Read the model definition and answer for the solid it produces. Units are mm, in the model's axes. A direction names the side the tool comes from. Give positions to 0.01 mm unless a question says otherwise; leave off trailing zeros. Order: outer loops, then holes, each group sorted by start corner. A loop starts at its lowest first (then second) coordinate and runs counter-clockwise, first axis right, second up. Notation, with made-up numbers: (5.5, -4) - (37.5, -4) arc R25 ccw to (37.5, 20) - close; hole circle Ø1 at (-25, -0.75). An arc over 180 degrees is marked (long way). Use a Markdown table: item, result. Add a question column.
1. Flat-ended cylindrical pins translate along their axes: P1, Ø6, axis at y = -3.5, z = 12.5, coming from the -X side; P2, Ø1.5, axis at x = 5, z = 33.5, coming from the -Y side; P3, Ø1.2, axis at y = 0, z = 114.5, coming from the +X side. Find the tip coordinate at first contact, or state that the pin passes through.
2. A cutting plane is placed at D-D on z = 97. Determine the outline of the cut face in (x, y), and give its area (3 significant figures).
3. For a pull along Y with two mould halves and no side action, classify faces 5 (the flat face through (0, 0, 90)), 6 (the flat face through (0, 0, 120)), 7 (the cylindrical face through (-1.5, -0.07, 44.37)), 8 (the flat face through (0, -2, 110)) as released by +Y, released by -Y, zero draft, split by the parting line, or undercut.
4. A cutting plane is placed at A-A on x = 0. Determine the outline of the cut face in (y, z), and give its area (3 significant figures).
5. Which of the six approach directions +Z, -Z, +X, -X, +Y, -Y give full straight-line access (tool end or side, diameter ignored) to faces 1 (the flat face through (2, 0, 110)), 2 (the flat face through (0, 2, 110)), 3 (the cylindrical face through (-1.08, -4.88, 51.33)), 4 (the flat face through (-2, 0, 110))?
6. Consider L1, parallel to Y at x = 0, z = 64.5; L2, parallel to Z at x = -6.5, y = 1. Determine where each line is inside the solid, lowest interval first.
7. A cutting plane is placed at C-C on z = 37.5. Determine the outline of the cut face in (x, y).
```python
from build123d import *

# Parameters (mm, degrees)
F0_R     = 7.5
F1_DEPTH = 4
F2_R     = 5
F3_DEPTH = 100
F4_W     = 4
F4_H     = 4
F5_DEPTH = 20
F6_R     = 1.5
F7_DEPTH = 90


with BuildPart() as f1:
    # F0 (on Top) → F1 (new body)
    with BuildSketch(Plane.XY):
        Circle(F0_R)
    extrude(amount=F1_DEPTH)

    # F2 (on Top) → F3 (join)
    with BuildSketch(Plane.XY):
        Circle(F2_R)
    extrude(amount=F3_DEPTH)

    # F4 (on face) → F5 (join)
    with BuildSketch(Plane.XY.offset(100)):
        Rectangle(F4_W, F4_H)
    extrude(amount=F5_DEPTH)

    # F6 (on face) → F7 (cut)
    with BuildSketch(Plane(origin=(0, 0, 0), x_dir=(1, 0, 0), z_dir=(0, 0, -1))):
        Circle(F6_R)
    extrude(amount=-F7_DEPTH, mode=Mode.SUBTRACT)


solid = f1.part
```
Output values:
| question | item | result |
|---|---|---|
| 1 | P1 | x = -4.97 |
| 1 | P2 | y = -2.63 |
| 1 | P3 | x = 2 |
| 2 | outline | circle Ø10 at (0, 0) |
| 2 | area | 78.5 mm² |
| 3 | face 5 | undercut |
| 3 | face 6 | zero draft |
| 3 | face 7 | undercut |
| 3 | face 8 | released by -Y |
| 4 | outline | (-7.5, 0) - (-1.5, 0) - (-1.5, 90) - (1.5, 90) - (1.5, 0) - (7.5, 0) - (7.5, 4) - (5, 4) - (5, 100) - (2, 100) - (2, 120) - (-2, 120) - (-2, 100) - (-5, 100) - (-5, 4) - (-7.5, 4) - close |
| 4 | area | 830 mm² |
| 5 | face 1 | +Z, +X, +Y, -Y |
| 5 | face 2 | +Z, +X, -X, +Y |
| 5 | face 3 | +Z |
| 5 | face 4 | +Z, -X, +Y, -Y |
| 6 | L1 | -5 to -1.5, 1.5 to 5 |
| 6 | L2 | 0 to 4 |
| 7 | outline | circle Ø10 at (0, 0); hole circle Ø3 at (0, 0) |
